For this review, use the dimensioned drawing (mm, ordinates from the lowest corner) and the shaded views. Round coordinates to 2 decimals unless told otherwise and drop trailing zeros. Order: outer loops, then holes, each group sorted by start corner. A loop starts at its lowest first (then second) coordinate and runs counter-clockwise, first axis right, second up. Notation, with made-up numbers: M 83.5,56 L 139.5,56 A4 ccw 139.5,61 Z; hole C 22,-4.75 d4. An arc over 180 degrees is marked long. Put each result on its own line as item: value.
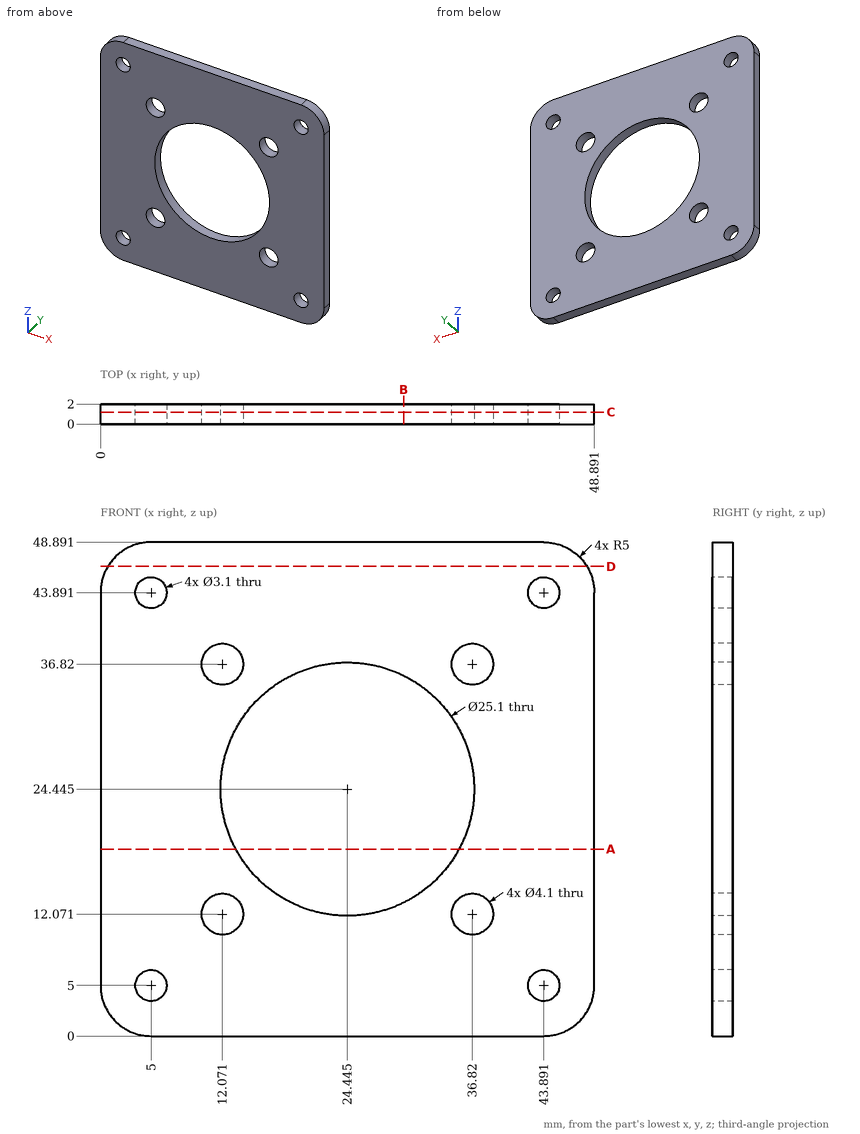
(1) To check wall thickness, follow L1, parallel to Z at x = 5, y = 1.1; L2, parallel to Z at x = 10.5, y = 1.3 (1 decimal); L3, parallel to X at y = 1.5, z = 4 (1 decimal). State the ranges of each line that lie inside material, in increasing order.
A:
L1: z = 0 to 3.45, 6.55 to 42.34, 45.44 to 48.89
L2: z = 0 to 10.8, 13.4 to 35.5, 38.1 to 48.9
L3: x = 0.1 to 3.8, 6.2 to 42.7, 45.1 to 48.8
(2) Insertion check: pin 1 Ø6.5 at (x, z) = (12.07, 36.82) entering from +Y. The pin has a flat end and moves straight along its axis. Give the tip position at first contact, or say it passes through.
A:
pin 1: stops at y = 2
(3) Add section D-D on z = 46.5. Give the boundary of the cut face in (x, y) (1 decimal).
A:
outline: M 0.7,0 L 48.2,0 L 48.2,2 L 0.7,2 Z
(4) Add section A-A on z = 18.5. Give the boundary of the cut face in (x, y).
A:
outline: M 0,0 L 13.39,0 L 13.39,2 L 0,2 Z; M 35.5,0 L 48.89,0 L 48.89,2 L 35.5,2 Z
(5) Add section B-B on x = 30. Give the boundary of the cut face in (y, z).
A:
outline: M 0,0 L 2,0 L 2,13.19 L 0,13.19 Z; M 0,35.7 L 2,35.7 L 2,48.89 L 0,48.89 Z
(6) Add section C-C on y = 1.2. State how many separate pieces and enclosed holes the cut face has, then the cut area to 3 significant figures.
A:
separate pieces: 1
enclosed holes: 9
area: 1,790 mm2
